from build123d import *

# Parameters (mm, degrees)
SKETCH1_W           = 11.938
SKETCH1_H           = 11.938
BOSS_EXTRUDE1_DEPTH = 213.106
SKETCH3_R           = 3.68046
BOSS_EXTRUDE3_DEPTH = 28.575
SKETCH5_R           = 9.137508411
CUT_EXTRUDE1_DEPTH  = 139.573
SKETCH6_W           = 7.0104
SKETCH6_H           = 7.0104
BOSS_EXTRUDE5_DEPTH = 12.7
SKETCH2_R           = 4.0005
CUT_EXTRUDE2_DEPTH  = 11.1125


with BuildPart() as part:
    # Sketch1 → Boss-Extrude1 (new body)
    with BuildSketch(Plane(origin=(0, 0, 0), x_dir=(1, 0, 0), z_dir=(0, 1, 0))):
        Rectangle(SKETCH1_W, SKETCH1_H)
    extrude(amount=BOSS_EXTRUDE1_DEPTH)

    # Sketch3 → Boss-Extrude3 (add)
    with BuildSketch(Plane(origin=(0, 0, 0), x_dir=(-1, 0, 0), z_dir=(0, -1, 0))):
        Circle(SKETCH3_R)
    extrude(amount=BOSS_EXTRUDE3_DEPTH)

    # Sketch5 → Cut-Extrude1 (cut)
    with BuildSketch(Plane(origin=(0, -28.575, 0), x_dir=(-1, 0, 0), z_dir=(0, -1, 0))):
        Circle(SKETCH5_R)
    extrude(amount=-CUT_EXTRUDE1_DEPTH, mode=Mode.SUBTRACT)

    # Sketch6 → Boss-Extrude5 (add)
    with BuildSketch(Plane(origin=(0, 110.998, 0), x_dir=(-1, 0, 0), z_dir=(0, -1, 0))):
        Rectangle(SKETCH6_W, SKETCH6_H)
    extrude(amount=BOSS_EXTRUDE5_DEPTH)

    # Sketch2 → Cut-Extrude2 (cut)
    with BuildSketch(Plane(origin=(0, 213.106, 0), x_dir=(1, 0, 0), z_dir=(0, 1, 0))):
        Circle(SKETCH2_R)
    extrude(amount=-CUT_EXTRUDE2_DEPTH, mode=Mode.SUBTRACT)


solid = part.part
The listing builds one solid part. Answer for the finished solid, in the listing's coordinates (mm). A direction names the side the tool comes from. Give positions to 0.01 mm unless a question says otherwise; leave off trailing zeros. Order: outer loops, then holes, each group sorted by start corner. A loop starts at its lowest first (then second) coordinate and runs counter-clockwise, first axis right, second up. Notation, with made-up numbers: (7.5, 53) - (35.5, 53) arc R34 ccw to (35.5, 83) - close; hole circle Ø4 at (49.25, -18). An arc over 180 degrees is marked (long way). One line per item, written item: value. Start each with the question number.
1) A tool of negligible diameter and unlimited length cuts with its end or side. For faces 4 (the face through (3.505, 105, 0)), 5 (the face through (0, 105, -3.505)), 6 (the face through (0, 105, 3.505)), 7 (the face through (0, 201.993, 0)), from which of +Z, -Z, +X, -X, +Y, -Y can it reach the whole face along a straight path? Write none if from no direction.
2) Given pin 1 Ø3.5 at (y, z) = (107, 0.5) entering from +X; pin 2 Ø2 at (x, y) = (-1, 103.5) entering from -Z, each flat-ended and moving along its own axis, determine where each tip first touches the part or whether it passes through.
3) A cutting plane is placed at B-B on x = 0. Give the vertices of the cut face in (y, z), then the cut area to 3 significant figures.
4) A cutting plane is placed at A-A on z = 0. Give the vertices of the cut face in (x, y).
5) The mould has two halves that part along X. Classify faces 1 (the face through (-0.9, 207.6, 3.9)), 2 (the face through (0, 161, -5.969)), 3 (the face through (-3.505, 105, 0)): released by +X, released by -X, zero draft, split by the parting line, or undercut.
6) Find the intervals of material crossed by L1, parallel to X at y = 209.5, z = 0; L2, parallel to Y at x = -0.25, z = 4.5, in increasing order.
Answer sheet:
1. face 4: +Z, -Z, +X, -Y
1. face 5: -Z, +X, -X, -Y
1. face 6: +Z, +X, -X, -Y
1. face 7: +Y
2. pin 1: stops at x = 3.51
2. pin 2: stops at z = -3.51
3. outline: (98.3, -3.51) - (111, -3.51) - (111, -5.97) - (213.11, -5.97) - (213.11, -4) - (201.99, -4) - (201.99, 4) - (213.11, 4) - (213.11, 5.97) - (111, 5.97) - (111, 3.51) - (98.3, 3.51) - close
3. area: 1,220 mm2
4. outline: (-5.97, 111) - (-3.51, 111) - (-3.51, 98.3) - (3.51, 98.3) - (3.51, 111) - (5.97, 111) - (5.97, 213.11) - (4, 213.11) - (4, 201.99) - (-4, 201.99) - (-4, 213.11) - (-5.97, 213.11) - close
5. face 1: undercut
5. face 2: zero draft
5. face 3: released by -X
6. L1: x = -5.97 to -4, 4 to 5.97
6. L2: y = 111 to 213.11
